Build history of the part. All positions in model axes, mm. A direction names the side the tool comes from. Give positions to 0.01 mm unless a question says otherwise; leave off trailing zeros. Loops run counter-clockwise (first coordinate to the right, second up) from the corner with the lowest first, then second, coordinate; pieces in that order, holes last. Notation, with made-up numbers: M 79,23.5 L 130,23.5 A19 ccw 130,37.5 Z; hole C 68.5,2.5 d9. An arc over 180 degrees is marked long. Answer as a JSON object with one key per item and string values. Group by question number.
1. Slice it at C-C (z = -6). List the corners of the cut face in (x, y), then the cut area to 3 significant figures.
2. Drill centre lines: line 1 along Y through (x, z) = (0, -10.05); line 2 along Z through (x, y) = (-3, -1.5); line 3 along X through (y, z) = (-1.5, 4.5). Where is each one in solid material? Low to high. Write a range as [from, to].
3. 3-axis set-ups, long thin cutter, end or side, ignore diameter. For faces 1 (the face through (-0.7, -2.5, -8.1)), 2 (the face through (0, 3, -13.5)), 3 (the face through (2.08, -1.5, -10.18)), 4 (the face through (7.74, 2.57, -4.59)), 5 (the face through (-0.26, 4.47, 11.68)): which of +Z, -Z, +X, -X, +Y, -Y reach the whole face in a straight line?
4. Mould opens along Z. For faces 6 (the face through (0, 3, 13.5)), 7 (the face through (0, 2.6, -7.6)), 8 (the face through (-0.7, 7.5, -8.1)) say: released by +Z, released by -Z, zero draft, split by the parting line, or undercut.
5. Slice it at D-D (x = -3). List the corners of the cut face in (y, z).
6. Drop flat-ended pins along their axis: pin 1 Ø2 at (x, y) = (6, 4.5) entering from -Z; pin 2 Ø6 at (y, z) = (-0.5, 8) entering from +X. Give the stop position or say it passes through.
7. Slice it at A-A (z = 0). List the corners of the cut face in (x, y).
8. Slice it at B-B (x = 0). List the corners of the cut face in (y, z).
from build123d import *

# Parameters (mm, degrees)
BOSS_EXTRUDE1_DEPTH      = 7.5
BOSS_EXTRUDE1_DEPTH_BACK = 2.5
SKETCH1_R                = 10.8
SKETCH1_R_2              = 7.6
BOSS_EXTRUDE2_DEPTH      = 13.5
BOSS_EXTRUDE2_DEPTH_BACK = 13.5
SKETCH2_R                = 2
SKETCH3_R                = 7.25
CUT_EXTRUDE1_DEPTH       = 14
SKETCH4_R                = 7
CUT_EXTRUDE2_DEPTH       = 10
FILLET2_R                = 1
CUT_EXTRUDE3_START       = -9.8
SKETCH5_R                = 4.5
SKETCH5_R_2              = 2
CUT_EXTRUDE3_DEPTH       = 9.5
CUT_EXTRUDE4_START       = 19.3
SKETCH6_R                = 4.5
SKETCH6_R_2              = 2
CUT_EXTRUDE4_DEPTH       = 9.5


with BuildPart() as part:
    # Sketch1 → Boss-Extrude1 (new, two sides: drawn at the far end of the back side and taken through both)
    with BuildSketch(Plane(origin=(0, 0, 0), x_dir=(1, 0, 0), z_dir=(0, 1, 0)).offset(-BOSS_EXTRUDE1_DEPTH_BACK)):
        with Locations(Location((0, 0, 0), (0, 0, 270))):
            Circle(SKETCH1_R)
        with Locations(Location((0, 0, 0), (0, 0, 270))):
            Circle(SKETCH1_R_2, mode=Mode.SUBTRACT)
    extrude(amount=BOSS_EXTRUDE1_DEPTH + BOSS_EXTRUDE1_DEPTH_BACK)

    # Sketch2 → Boss-Extrude2 (add, two sides: drawn at the far end of the back side and taken through both)
    with BuildSketch(Plane.XY.offset(-BOSS_EXTRUDE2_DEPTH_BACK)):
        with Locations((0, 2.488781623)):
            Circle(SKETCH2_R)
    extrude(amount=BOSS_EXTRUDE2_DEPTH + BOSS_EXTRUDE2_DEPTH_BACK)

    # Sketch3 → Cut-Extrude1 (cut)
    with BuildSketch(Plane(origin=(0, 7.5, 0), x_dir=(1, 0, 0), z_dir=(0, 1, 0))):
        Circle(SKETCH3_R)
    extrude(amount=-CUT_EXTRUDE1_DEPTH, mode=Mode.SUBTRACT)

    # Sketch4 → Cut-Extrude2 (cut)
    with BuildSketch(Plane(origin=(0, 7.5, 0), x_dir=(1, 0, 0), z_dir=(0, 1, 0))):
        with BuildLine():
            ThreePointArc((-1.274588785, 8.908659182), (0, 7.6), (1.274588785, 8.908659182))
            ThreePointArc((1.274588785, 8.908659182), (7.793689033, 4.499688461), (8.352419558, -3.350503324))
            ThreePointArc((8.352419558, -3.350503324), (6.581793069, -3.8), (7.077830773, -5.558155858))
            ThreePointArc((7.077830773, -5.558155858), (0, -8.999376922), (-7.077830773, -5.558155858))
            ThreePointArc((-7.077830773, -5.558155858), (-6.581793069, -3.8), (-8.352419558, -3.350503324))
            ThreePointArc((-8.352419558, -3.350503324), (-7.793689033, 4.499688461), (-1.274588785, 8.908659182))
        make_face()
        Circle(SKETCH4_R, mode=Mode.SUBTRACT)
    extrude(amount=-CUT_EXTRUDE2_DEPTH, mode=Mode.SUBTRACT)

    # Fillet2
    fillet2_edges = [part.edges().sort_by_distance(p)[0] for p in [
        (-8.352419558, 2.5, 3.350503324),
        (-1.274588785, 2.5, -8.908659182),
        (1.274588785, 2.5, -8.908659182),
        (8.352419558, 2.5, 3.350503324),
        (7.077830773, 2.5, 5.558155858),
        (-7.077830773, 2.5, 5.558155858),
    ]]
    fillet(fillet2_edges, radius=FILLET2_R)

    # Sketch5 → Cut-Extrude3 (cut)
    with BuildSketch(Plane.XY.offset(CUT_EXTRUDE3_START)):
        with Locations((0, 2.488781623)):
            Circle(SKETCH5_R)
        with Locations((0, 2.488781623)):
            Circle(SKETCH5_R_2, mode=Mode.SUBTRACT)
    extrude(amount=-CUT_EXTRUDE3_DEPTH, mode=Mode.SUBTRACT)

    # Sketch6 → Cut-Extrude4 (cut)
    with BuildSketch(Plane.XY.offset(CUT_EXTRUDE4_START)):
        with Locations((0, 2.488781623)):
            Circle(SKETCH6_R)
        with Locations((0, 2.488781623)):
            Circle(SKETCH6_R_2, mode=Mode.SUBTRACT)
    extrude(amount=-CUT_EXTRUDE4_DEPTH, mode=Mode.SUBTRACT)


solid = part.part
Established:
{
 "1": {"outline": "M -8.98,-2.5 L -6.71,-2.5 L -6.71,7.5 L -8.98,7.5 Z; M 6.71,-2.5 L 8.98,-2.5 L 8.98,7.5 L 6.71,7.5 Z", "area": "45.5 mm^2"},
 "2": {"line 1": "y = [-2.5, -2.01], [0.49, 4.49], [6.99, 7.5]", "line 2": "z = [-10.37, -8.48], [8.48, 10.37]", "line 3": "x = [-9.82, -6.41], [6.41, 9.82]"},
 "3": {"face 1": "+Z, -Z, +X, -X, -Y", "face 2": "-Z, +X, -X, +Y, -Y", "face 3": "-Z", "face 4": "+Y, -Y", "face 5": "+Z"},
 "4": {"face 6": "released by +Z", "face 7": "undercut", "face 8": "zero draft"},
 "5": {"outline": "M -2.5,-10.37 L -0.87,-10.37 L -0.87,-9.8 L 5.84,-9.8 L 5.84,-10.37 L 7.5,-10.37 L 7.5,-8.48 L -2.5,-8.48 Z; M -2.5,8.48 L 7.5,8.48 L 7.5,10.37 L 5.84,10.37 L 5.84,9.8 L -0.87,9.8 L -0.87,10.37 L -2.5,10.37 Z"},
 "6": {"pin 1": "stops at z = -9.57", "pin 2": "stops at x = 9.57"},
 "7": {"outline": "M -10.8,-2.5 L -9,-2.5 L -9,7.5 L -10.8,7.5 Z; M 9,-2.5 L 10.8,-2.5 L 10.8,7.5 L 9,7.5 Z"},
 "8": {"outline": "M -2.5,-10.8 L -2.01,-10.8 L -2.01,-9.8 L 0.49,-9.8 L 0.49,-13.5 L 4.49,-13.5 L 4.49,-9.8 L 6.99,-9.8 L 6.99,-10.8 L 7.5,-10.8 L 7.5,-7.6 L -2.5,-7.6 Z; M -2.5,9 L 7.5,9 L 7.5,10.8 L 6.99,10.8 L 6.99,9.8 L 4.49,9.8 L 4.49,13.5 L 0.49,13.5 L 0.49,9.8 L -2.01,9.8 L -2.01,10.8 L -2.5,10.8 Z"}
}
